Check sheet for the drawn part. Datum: minimum x, y, z corner. Units: mm. A direction names the side the tool comes from. Round coordinates to 2 decimals unless told otherwise and drop trailing zeros. Order: outer loops, then holes, each group sorted by start corner. A loop starts at its lowest first (then second) coordinate and runs counter-clockwise, first axis right, second up.
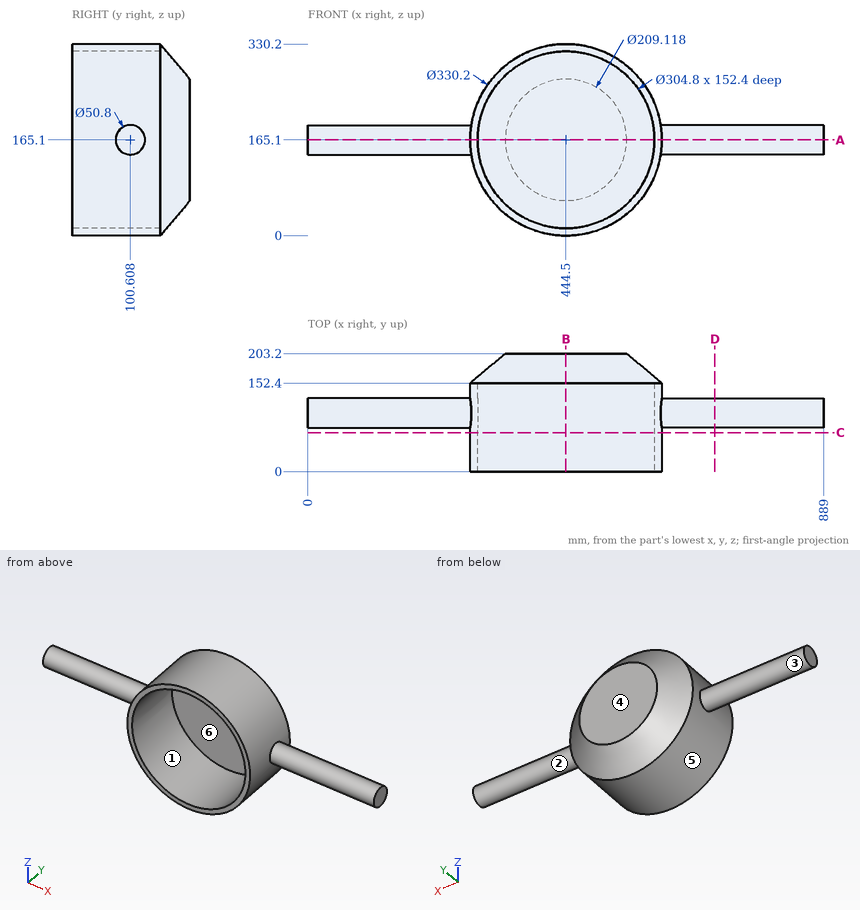
1) Sectioned sample at B-B on x = 444.5. Record the cut outline in (y, z).
2) Gauge pin test, flat ends, axial feed: pin 1 (2 mm diameter, centred on x = 352.5, y = 61.5, fed in from -Z); pin 2 (6 mm diameter, centred on x = 162.5, y = 105, fed in from +Z); pin 3 (3 mm diameter, centred on x = 143.5, y = 76, fed in from -Z) (1 decimal). Record the tip position at first contact, or that the pin passes through.
3) Scan lines: line 1 (Z direction, x = 444.5, y = 66.5); line 2 (X direction, y = 56, z = 165); line 3 (X direction, y = 100, z = 165). Record each from-to range of solid material in increasing order.
4) Sectioned sample at C-C on y = 67. Record the cut outline in (x, z), and give its area (3 significant figures).
5) Sectioned sample at A-A on z = 165.1. Record the cut outline in (x, y), and give its area (3 significant figures).
6) Sectioned sample at D-D on x = 701. Record the cut outline in (y, z), and give its area (3 significant figures).
7) Set-up check for the marked faces 1, 2 and 3: record each of +Z, -Z, +X, -X, +Y, -Y from which the full face is reachable in a straight line by a thin tool's end or side.
8) Draft check along Z on the marked faces 4, 5 and 6. Enter one of: pulls with the +Z half, pulls with the -Z half, needs draft (parallel to the pull), parting line crosses it, or undercut.
Values found:
1. outline: (0, 0) - (152.4, 0) - (203.2, 60.54) - (203.2, 269.66) - (152.4, 330.2) - (0, 330.2) - (0, 317.5) - (152.4, 317.5) - (152.4, 12.7) - (0, 12.7) - close
2. pin 1: stops at z = 27.34
2. pin 2: stops at z = 190.46
2. pin 3: stops at z = 154.6
3. line 1: z = 0 to 12.7, 317.5 to 330.2
3. line 2: x = 279.4 to 292.1, 596.9 to 609.6
3. line 3: x = 0 to 292.1, 596.9 to 889
4. outline: circle Ø330.2 at (444.5, 165.1); hole circle Ø304.8 at (444.5, 165.1)
4. area: 12,700 mm2
5. outline: (0, 75.21) - (279.4, 75.21) - (279.4, 0) - (292.1, 0) - (292.1, 152.4) - (596.9, 152.4) - (596.9, 0) - (609.6, 0) - (609.6, 75.21) - (889, 75.21) - (889, 126.01) - (609.6, 126.01) - (609.6, 152.4) - (549.06, 203.2) - (339.94, 203.2) - (279.4, 152.4) - (279.4, 126.01) - (0, 126.01) - close
5. area: 46,000 mm2
6. outline: circle Ø50.8 at (100.61, 165.1)
6. area: 2,030 mm2
7. face 1: -Y
7. face 2: +X
7. face 3: -X
8. face 4: needs draft
8. face 5: parting line crosses it
8. face 6: undercut
